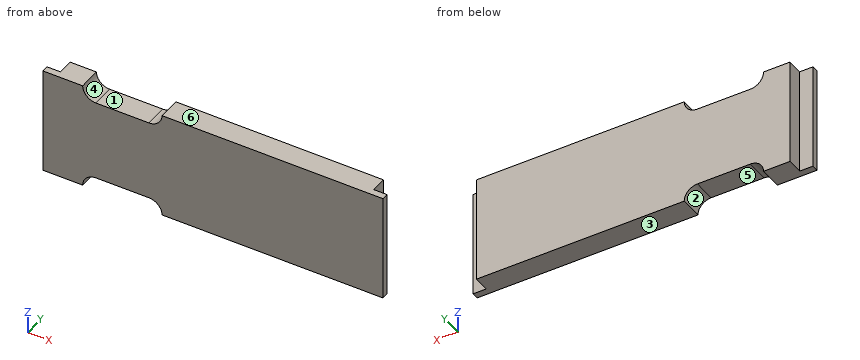
from build123d import *

# Parameters (mm, degrees)
PAD_DEPTH    = 40.64
POCKET_DEPTH = 21


with BuildPart() as part:
    # Sketch → Pad (new body)
    with BuildSketch(Plane.XY):
        Polygon((0, 0), (0, 2.51), (5, 2.51), (4.999966, 8.51), (123.5, 8.51), (123.5, 2.51), (128.5, 2.51), (128.5, 0), align=None)
    extrude(amount=PAD_DEPTH)

    # Sketch002 → Pocket (cut)
    with BuildSketch(Plane.XZ):
        with BuildLine():
            ThreePointArc((20, 5), (15, 0), (20, -5))
            Line((20, -5), (40, -5))
            ThreePointArc((40, -5), (45, 0), (40, 5))
            Line((40, 5), (20, 5))
        make_face()
        with BuildLine():
            ThreePointArc((20, 45.64), (15, 40.64), (20, 35.64))
            Line((20, 35.64), (40, 35.64))
            ThreePointArc((40, 35.64), (45, 40.64), (40, 45.64))
            Line((40, 45.64), (20, 45.64))
        make_face()
    extrude(amount=-POCKET_DEPTH, mode=Mode.SUBTRACT)


solid = part.part
Input: part model. Units: mm. Frame: model coordinates. Face numbers are marked on the shaded views. A direction names the side the tool comes from. Coordinates: 2 decimals unless noted, no trailing zeros. Loops run counter-clockwise (first coordinate to the right, second up) from the corner with the lowest first, then second, coordinate; pieces in that order, holes last.
Q1. Cut plane B-B (y = 6.75). Output: boundary loops of the cut face in (x, z).
Q2. Cut plane A-A (z = 3.5). Output: boundary loops of the cut face in (x, y), then the cut area to 3 significant figures.
Q3. Draft query along X for the marked faces 1, 2 and 3. Return one class per face: +X half, -X half, draft (parallel to the pull), parting line (faces both ways), or undercut.
Q4. Cut plane C-C (z = 11.5). Output: boundary loops of the cut face in (x, y).
Q5. Set-up query: the marked faces 4, 5 and 6. Return all of +Z, -Z, +X, -X, +Y, -Y with unobstructed straight access to the full face (end or side cutting, diameter ignored); none if empty.
Q6. Contact query for flat-ended pins moving along their axis: pin 1 (4 mm diameter, centred on x = 127, z = 16, fed in from +Y); pin 2 (4.5 mm diameter, centred on x = 30.5, y = 3.5, fed in from +Z); pin 3 (4 mm diameter, centred on x = 38.5, y = 1.5, fed in from -Z). Output: stop coordinate, or through.
Q7. Cut plane D-D (x = 37). Output: boundary loops of the cut face in (y, z).
Q8. Material intervals for line 1 (X direction, y = 4.75, z = 6); line 2 (Z direction, x = 29, y = 5); line 3 (X direction, y = 3.25, z = 3), sorted ascending.
Working result:
1. outline: (5, 0) - (15, 0) arc R5 cw to (20, 5) - (40, 5) arc R5 cw to (45, 0) - (123.5, 0) - (123.5, 40.64) - (45, 40.64) arc R5 cw to (40, 35.64) - (20, 35.64) arc R5 cw to (15, 40.64) - (5, 40.64) - close
2. outline: (0, 0) - (16.43, 0) - (16.43, 8.51) - (5, 8.51) - (5, 2.51) - (0, 2.51) - close; (43.57, 0) - (128.5, 0) - (128.5, 2.51) - (123.5, 2.51) - (123.5, 8.51) - (43.57, 8.51) - close
2. area: 803 mm2
3. face 1: undercut
3. face 2: undercut
3. face 3: draft
4. outline: (0, 0) - (128.5, 0) - (128.5, 2.51) - (123.5, 2.51) - (123.5, 8.51) - (5, 8.51) - (5, 2.51) - (0, 2.51) - close
5. face 4: +Z, +Y, -Y
5. face 5: -Z, +Y, -Y
5. face 6: +Z, +X, -X, +Y, -Y
6. pin 1: stops at y = 2.51
6. pin 2: stops at z = 35.64
6. pin 3: stops at z = 4.97
7. outline: (0, 5) - (8.51, 5) - (8.51, 35.64) - (0, 35.64) - close
8. line 1: x = 5 to 123.5
8. line 2: z = 5 to 35.64
8. line 3: x = 5 to 16, 44 to 123.5
